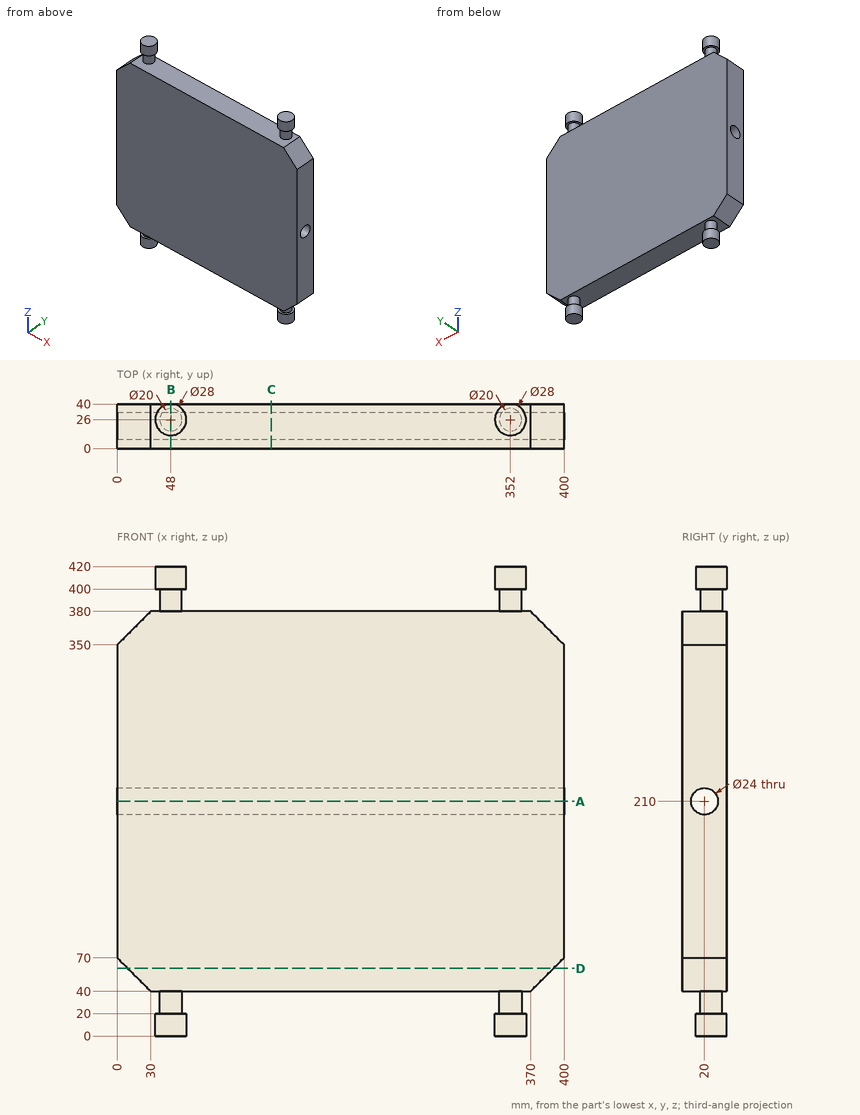
Drawing for the job (mm, zero at the part's lowest x, y, z). Round coordinates to 2 decimals unless told otherwise and drop trailing zeros. Write each loop counter-clockwise with the first axis right and the second up, starting at its lowest first coordinate (ties: lowest second). Pieces come first, ordered by that corner, then holes.
Item 1: Band-saw the part on A-A on z = 210. Write the cut outline in (x, y), then the cut area to 3 significant figures.
Filled in:
outline: (0, 0) - (400, 0) - (400, 8) - (0, 8) - close; (0, 32) - (400, 32) - (400, 40) - (0, 40) - close
area: 6,400 mm2
Item 2: Band-saw the part on B-B on x = 48. Write the cut outline in (y, z), then the cut area to 3 significant figures.
Filled in:
outline: (0, 40) - (16, 40) - (16, 20) - (12, 20) - (12, 0) - (40, 0) - (40, 20) - (36, 20) - (36, 40) - (40, 40) - (40, 380) - (36, 380) - (36, 400) - (40, 400) - (40, 420) - (12, 420) - (12, 400) - (16, 400) - (16, 380) - (0, 380) - close; hole circle Ø24 at (20, 210)
area: 15,100 mm2
Item 3: Drill centre lines: L1, parallel to Y at x = 135, z = 210; L2, parallel to Z at x = 91, y = 21.5; L3, parallel to Z at x = 216, y = 28. Where is each one in solid material? Low to high.
Filled in:
L1: y = 0 to 8, 32 to 40
L2: z = 40 to 198.09, 221.91 to 380
L3: z = 40 to 201.06, 218.94 to 380
Item 4: Drop flat-ended pins along their axis: pin 1 Ø4 at (x, y) = (206, 35.5) entering from -Z; pin 2 Ø2 at (x, y) = (110, 12.5) entering from +Z; pin 3 Ø5 at (y, z) = (23.5, 218) entering from +X. Give the stop position or say it passes through.
Filled in:
pin 1: stops at z = 40
pin 2: stops at z = 380
pin 3: passes through
Item 5: Band-saw the part on D-D on z = 60.5. Write the cut outline in (x, y).
Filled in:
outline: (9.5, 0) - (390.5, 0) - (390.5, 40) - (9.5, 40) - close
Item 6: Band-saw the part on C-C on x = 138. Write the cut outline in (y, z).
Filled in:
outline: (0, 40) - (40, 40) - (40, 380) - (0, 380) - close; hole circle Ø24 at (20, 210)
